Work out the finished part from the listing and answer in its coordinate system (mm). Face numbers are marked on the shaded views. A direction names the side the tool comes from. Coordinates: 2 decimals unless noted, no trailing zeros. Loops run counter-clockwise (first coordinate to the right, second up) from the corner with the lowest first, then second, coordinate; pieces in that order, holes last.
```python
from build123d import *

# Parameters (mm, degrees)
SKETCH1_W           = 15
SKETCH1_H           = 25
BOSS_EXTRUDE1_DEPTH = 25


with BuildPart() as part:
    # Sketch1 → Boss-Extrude1 (new body)
    with BuildSketch(Plane.XY):
        with BuildLine():
            Line((0, -20), (0, 0))
            Line((0, 0), (-5, 0))
            ThreePointArc((-5, 0), (-15, -10), (-5, -20))
            Line((-5, -20), (0, -20))
        make_face()
        with Locations((7.5, -12.5)):
            Rectangle(SKETCH1_W, SKETCH1_H)
    extrude(amount=BOSS_EXTRUDE1_DEPTH)


solid = part.part
```
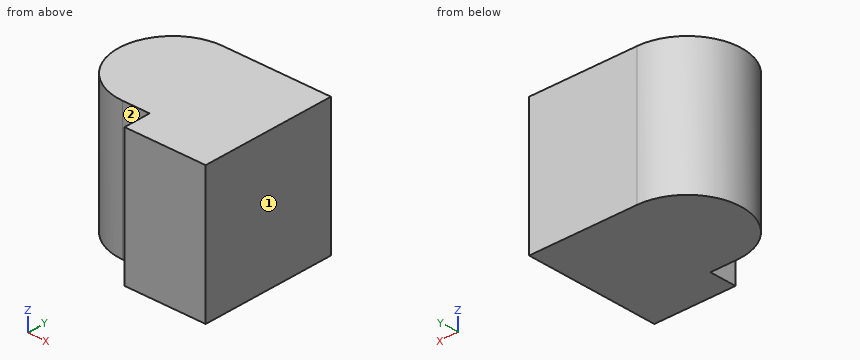
1. A cutting plane is placed at C-C, the plane x = -0.75. Give the vertices of the cut face in (y, z).
2. Straight lines are drawn through the part: probe 1 along X at (y, z) = (-23.25, 15.5); probe 2 along X at (y, z) = (-1.75, 14.75); probe 3 along Y at (x, z) = (-9, 21.25). For each, find the intervals that lie inside material, in ascending order.
3. A cutting plane is placed at B-B, the plane z = 11.75. Give the vertices of the cut face in (x, y).
4. Each of these flat-tipped pins is pushed along its axis until it touches: P1, Ø5.5, axis at x = -3, z = 13.5, coming from the -Y side; P2, Ø1.5, axis at y = -23.5, z = 11, coming from the -X side. Where does it stop, or does it pass through?
5. A cutting plane is placed at A-A, the plane y = -21. Give the vertices of the cut face in (x, z).
6. For the marked faces 1 and 2, determine the directions among +Z, -Z, +X, -X, +Y, -Y from which every point of the face is accessible in a straight line to the end or side of a thin tool.
Answers below:
1. outline: (-20, 0) - (0, 0) - (0, 25) - (-20, 25) - close
2. probe 1: x = 0 to 15
2. probe 2: x = -10.65 to 15
2. probe 3: y = -19.17 to -0.83
3. outline: (-5, -20) - (0, -20) - (0, -25) - (15, -25) - (15, 0) - (-5, 0) arc R10 ccw to start
4. P1: stops at y = -20
4. P2: stops at x = 0
5. outline: (0, 0) - (15, 0) - (15, 25) - (0, 25) - close
6. face 1: +Z, -Z, +X, +Y, -Y
6. face 2: +Z, -Z, -X, -Y
